Build history of the part. All positions in model axes, mm. Face numbers are marked on the shaded views. A direction names the side the tool comes from. Coordinates: 2 decimals unless noted, no trailing zeros. Order: outer loops, then holes, each group sorted by start corner. A loop starts at its lowest first (then second) coordinate and runs counter-clockwise, first axis right, second up. Notation, with made-up numbers: (25.5, 50) - (45.5, 50) arc R14 cw to (45.5, 75) - close; hole circle Ø6 at (-12, -39.5). An arc over 180 degrees is marked (long way). Return JSON: item names as keys, results as strings.
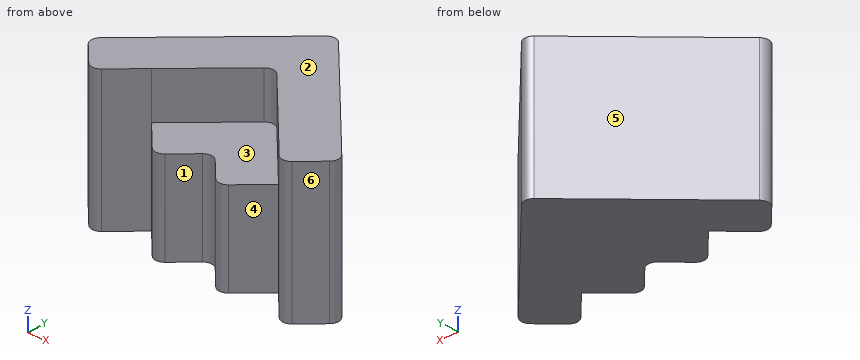
from build123d import *

# Parameters (mm, degrees)
F1_DEPTH = 25.4
F3_DEPTH = 25.4
F5_DEPTH = 50.8
F6_R     = 5.08
F7_R     = 5.08
F8_R     = 5.08
F9_R     = 5.08
F10_R    = 5.08
F11_R    = 5.08
F12_R    = 5.08
F13_R    = 5.08
F14_R    = 5.08


with BuildPart() as f1:
    # F0 (on Top) → F1 (new body)
    with BuildSketch(Plane.XY):
        Polygon((69.5630275399, -20.6164596444), (0, 53.434503884), (-74.0509635284, -16.1285236559), (-56.6602066435, -34.641264538), (-38.1474657613, -17.250507653), (-20.7567088764, -35.7632485351), (-2.2439679943, -18.3724916501), (15.1467888907, -36.8852325322), (33.6595297728, -19.4944756473), (51.0502866578, -38.0072165294), align=None)
    extrude(amount=F1_DEPTH)

    # F2 (on face) → F3 (join)
    with BuildSketch(Plane.XY.offset(25.4)):
        Polygon((-1.1219839971, 17.5310061169), (-38.1474657613, -17.250507653), (-20.7567088764, -35.7632485351), (-2.2439679943, -18.3724916501), (15.1467888907, -36.8852325322), (33.6595297728, -19.4944756473), align=None)
    extrude(amount=F3_DEPTH)

    # F4 (on face) → F5 (join)
    with BuildSketch(Plane.XY.offset(25.4)):
        Polygon((33.6595297728, -19.4944756473), (51.0502866578, -38.0072165294), (69.5630275399, -20.6164596444), (0, 53.434503884), (-74.0509635284, -16.1285236559), (-56.6602066435, -34.641264538), (-38.1474657613, -17.250507653), (-1.1219839971, 17.5310061169), align=None)
    extrude(amount=F5_DEPTH)

    # F6
    f6_edges = [f1.edges().sort_by_distance(p)[0] for p in [
        (-1.121984, 17.531006, 63.5),
    ]]
    fillet(f6_edges, radius=F6_R)

    # F7
    f7_edges = [f1.edges().sort_by_distance(p)[0] for p in [
        (-2.243968, -18.372492, 25.4),
    ]]
    fillet(f7_edges, radius=F7_R)

    # F8
    f8_edges = [f1.edges().sort_by_distance(p)[0] for p in [
        (15.146789, -36.885233, 25.4),
    ]]
    fillet(f8_edges, radius=F8_R)

    # F9
    f9_edges = [f1.edges().sort_by_distance(p)[0] for p in [
        (-20.756709, -35.763249, 25.4),
    ]]
    fillet(f9_edges, radius=F9_R)

    # F10
    f10_edges = [f1.edges().sort_by_distance(p)[0] for p in [
        (0, 53.434504, 38.1),
    ]]
    fillet(f10_edges, radius=F10_R)

    # F11
    f11_edges = [f1.edges().sort_by_distance(p)[0] for p in [
        (-74.050964, -16.128524, 38.1),
    ]]
    fillet(f11_edges, radius=F11_R)

    # F12
    f12_edges = [f1.edges().sort_by_distance(p)[0] for p in [
        (69.563028, -20.61646, 38.1),
    ]]
    fillet(f12_edges, radius=F12_R)

    # F13
    f13_edges = [f1.edges().sort_by_distance(p)[0] for p in [
        (-56.660207, -34.641265, 38.1),
    ]]
    fillet(f13_edges, radius=F13_R)

    # F14
    f14_edges = [f1.edges().sort_by_distance(p)[0] for p in [
        (51.050287, -38.007217, 38.1),
    ]]
    fillet(f14_edges, radius=F14_R)


solid = f1.part
1. Cut at A-A on z = 34. Give the cut face in (x, y), plus the area to 3 significant figures.
Check values:
{"outline": "(-70.57, -19.83) - (-60.14, -30.94) arc R5.08 ccw to (-52.96, -31.16) - (-38.15, -17.25) - (-24.23, -32.06) arc R5.08 ccw to (-17.05, -32.29) - (-5.95, -21.85) arc R5.08 cw to (1.23, -22.08) - (11.67, -33.18) arc R5.08 ccw to (18.85, -33.41) - (33.66, -19.49) - (47.57, -34.3) arc R5.08 ccw to (54.75, -34.53) - (65.86, -24.09) arc R5.08 ccw to (66.08, -16.91) - (3.48, 49.73) arc R5.08 ccw to (-3.7, 49.96) - (-70.35, -12.65) arc R5.08 ccw to start", "area": "6,420 mm²"}
2. Cut at B-B on y = 7. Give the cut face in (x, z), plus the area to 3 significant figures.
Check values:
{"outline": "(-49.43, 0) - (43.62, 0) - (43.62, 76.2) - (8.77, 76.2) - (8.77, 50.8) - (-12.33, 50.8) - (-12.33, 76.2) - (-49.43, 76.2) - close", "area": "6,550 mm²"}
3. Probe L1, parallel to X at y = -28.5, z = 22.5; L2, parallel to X at y = -29, z = 42.5; L3, parallel to X at y = -9, z = 54. List the from-to ranges inside material, lowest first.
Check values:
{"L1": "-62.43 to -50.12, -27.58 to -13.02, 7.27 to 24.07, 42.12 to 61.17", "L2": "-61.96 to -50.65, -27.11 to -13.56, 7.74 to 23.54, 42.59 to 60.64", "L3": "-66.46 to -29.36, 23.8 to 58.65"}
4. Mould opens along X. For the marked faces 4, 5 and 6 say: pulls with the +X half, pulls with the -X half, needs draft (parallel to the pull), parting line crosses it, or undercut.
Check values:
{"face 4": "undercut", "face 5": "pulls with the -X half", "face 6": "pulls with the +X half"}
5. Cut at D-D on z = 54. Give the cut face in (x, y).
Check values:
{"outline": "(-70.57, -19.83) - (-60.14, -30.94) arc R5.08 ccw to (-52.96, -31.16) - (-4.82, 14.05) arc R5.08 cw to (2.36, 13.83) - (47.57, -34.3) arc R5.08 ccw to (54.75, -34.53) - (65.86, -24.09) arc R5.08 ccw to (66.08, -16.91) - (3.48, 49.73) arc R5.08 ccw to (-3.7, 49.96) - (-70.35, -12.65) arc R5.08 ccw to start"}
6. Tool access for the marked faces 1, 2 and 3: list every direction of +Z, -Z, +X, -X, +Y, -Y with a clear straight run to the whole face (end or side of a thin tool).
Check values:
{"face 1": "+Z, -Z, -Y", "face 2": "+Z, +X, -X, +Y, -Y", "face 3": "+Z, -Y"}
7. Drop flat-ended pins along their axis: pin 1 (6 mm diameter, centred on x = -18, z = 51, fed in from -Y); pin 2 (1 mm diameter, centred on y = -23, z = 41.5, fed in from +X); pin 3 (10 mm diameter, centred on x = 31, z = 34.5, fed in from -Y). Give the stop position or say it passes through.
Check values:
{"pin 1": "y = -33.66", "pin 2": "x = 67", "pin 3": "y = -26.69"}
8. Cut at C-C on x = -9. Give the cut face in (y, z).
Check values:
{"outline": "(-24.72, 0) - (44.98, 0) - (44.98, 76.2) - (10.13, 76.2) - (10.13, 50.8) - (-24.72, 50.8) - close"}
